The model under review builds one solid part; all positions refer to its coordinate system, in mm. Round coordinates to 2 decimals unless told otherwise and drop trailing zeros. Loops run counter-clockwise (first coordinate to the right, second up) from the corner with the lowest first, then second, coordinate; pieces in that order, holes last. Notation, with made-up numbers: (-37.5, 45.25) -> (-26.5, 45.25) arc R25 cw to (-26.5, 83.25) -> close; hole circle Ø1 at (28, 14.5). An arc over 180 degrees is marked (long way). Use a Markdown table: item, result. Add a question column.
1) Consider section A-A on z = 76.5. Give the boundary of the cut face in (x, y), plus the area to 3 significant figures.
2) Consider section C-C on x = -79. Give the boundary of the cut face in (y, z), plus the area to 3 significant figures.
3) Consider section B-B on y = 0.8. State how many separate pieces and enclosed holes the cut face has, plus the area to 3 significant figures.
4) Wall thickness on probe 1 along X at (y, z) = (1.95, -115.5); probe 2 along Z at (x, y) = (101.6, 2.7); probe 3 along X at (y, z) = (4.45, 19): over which ranges is each line inside the solid? List them lowest first.
5) Insertion check: pin 1 (1 mm diameter, centred on y = 3, z = 3, fed in from -X); pin 2 (2.5 mm diameter, centred on y = 3, z = -164.5, fed in from +X); pin 3 (2.5 mm diameter, centred on y = 3.5, z = -164, fed in from -X). Each pin has a flat end and moves straight along its axis. Give the tip position at first contact, or say it passes through.
from build123d import *

# Parameters (mm, degrees)
SKETCH1_R           = 177
SKETCH1_R_2         = 1.6
SKETCH1_R_3         = 2.2479
SKETCH1_R_4         = 2.000000064
SKETCH1_R_5         = 1.3
SKETCH1_R_6         = 1.29999994
SKETCH1_W           = 6.15
SKETCH1_H           = 6.15
SKETCH1_W_2         = 30
SKETCH1_H_2         = 80
SKETCH1_W_3         = 6.35
SKETCH1_H_3         = 3.175
BOSS_EXTRUDE1_DEPTH = 4.7625
SKETCH2_R           = 1.599999975
CUT_EXTRUDE1_DEPTH  = 251.361102023
SKETCH3_R           = 1.3
SKETCH3_R_2         = 1.29999994
SKETCH3_W           = 6.15
SKETCH3_H           = 6.15
CUT_EXTRUDE2_DEPTH  = 251.361102023


with BuildPart() as part:
    # Sketch1 → Boss-Extrude1 (new body)
    with BuildSketch(Plane(origin=(0, 0, 0), x_dir=(1, 0, 0), z_dir=(0, 1, 0))):
        with Locations(Location((0, 0, 0), (0, 0, 90))):
            Circle(SKETCH1_R)
        with Locations(Location((-150.65, 25.4, 0), (0, 0, 90))):
            Circle(SKETCH1_R_2, mode=Mode.SUBTRACT)
        with Locations(Location((-150.65, -25.4, 0), (0, 0, 90))):
            Circle(SKETCH1_R_2, mode=Mode.SUBTRACT)
        with Locations(Location((150.65, 25.4, 0), (0, 0, 90))):
            Circle(SKETCH1_R_2, mode=Mode.SUBTRACT)
        with Locations(Location((150.65, -25.4, 0), (0, 0, 90))):
            Circle(SKETCH1_R_2, mode=Mode.SUBTRACT)
        with Locations(Location((-107.95, 25.4, 0), (0, 0, 90))):
            Circle(SKETCH1_R_2, mode=Mode.SUBTRACT)
        with Locations(Location((-107.95, -25.4, 0), (0, 0, 90))):
            Circle(SKETCH1_R_2, mode=Mode.SUBTRACT)
        with Locations(Location((107.95, 25.4, 0), (0, 0, 90))):
            Circle(SKETCH1_R_2, mode=Mode.SUBTRACT)
        with Locations(Location((107.95, -25.4, 0), (0, 0, 90))):
            Circle(SKETCH1_R_2, mode=Mode.SUBTRACT)
        with Locations(Location((-53.7, 114.3, 0), (0, 0, 90))):
            Circle(SKETCH1_R_2, mode=Mode.SUBTRACT)
        with Locations(Location((38.8, 114.3, 0), (0, 0, 90))):
            Circle(SKETCH1_R_2, mode=Mode.SUBTRACT)
        with Locations(Location((-53.7, 35.8, 0), (0, 0, 90))):
            Circle(SKETCH1_R_2, mode=Mode.SUBTRACT)
        with Locations(Location((38.8, 35.8, 0), (0, 0, 90))):
            Circle(SKETCH1_R_2, mode=Mode.SUBTRACT)
        with Locations(Location((-101.6, -101.6, 0), (0, 0, 90))):
            Circle(SKETCH1_R_3, mode=Mode.SUBTRACT)
        with Locations(Location((101.6, -101.6, 0), (0, 0, 90))):
            Circle(SKETCH1_R_3, mode=Mode.SUBTRACT)
        with Locations(Location((-101.6, 101.6, 0), (0, 0, 90))):
            Circle(SKETCH1_R_3, mode=Mode.SUBTRACT)
        with Locations(Location((101.6, 101.6, 0), (0, 0, 90))):
            Circle(SKETCH1_R_3, mode=Mode.SUBTRACT)
        with Locations(Location((-20, -142.687006289, 0), (0, 0, 90))):
            Circle(SKETCH1_R_4, mode=Mode.SUBTRACT)
        with Locations(Location((20, -142.687006289, 0), (0, 0, 90))):
            Circle(SKETCH1_R_4, mode=Mode.SUBTRACT)
        with Locations(Location((-20, 151.719279026, 0), (0, 0, 90))):
            Circle(SKETCH1_R_4, mode=Mode.SUBTRACT)
        with Locations(Location((20, 151.719279026, 0), (0, 0, 90))):
            Circle(SKETCH1_R_4, mode=Mode.SUBTRACT)
        with Locations(Location((-10.125, -171.45, 0), (0, 0, 90))):
            Circle(SKETCH1_R_5, mode=Mode.SUBTRACT)
        with Locations(Location((10.125, -171.45, 0), (0, 0, 90))):
            Circle(SKETCH1_R_6, mode=Mode.SUBTRACT)
        with Locations(Location((171.45, -10.125, 0), (0, 0, 90))):
            Circle(SKETCH1_R_5, mode=Mode.SUBTRACT)
        with Locations(Location((171.45, 10.125, 0), (0, 0, 90))):
            Circle(SKETCH1_R_5, mode=Mode.SUBTRACT)
        with Locations(Location((-171.45, -10.125, 0), (0, 0, 90))):
            Circle(SKETCH1_R_5, mode=Mode.SUBTRACT)
        with Locations(Location((-171.45, 10.125, 0), (0, 0, 90))):
            Circle(SKETCH1_R_5, mode=Mode.SUBTRACT)
        with Locations((171.45, 4.26)):
            Rectangle(SKETCH1_W, SKETCH1_H, mode=Mode.SUBTRACT)
        with Locations((-129.3, 0)):
            Rectangle(SKETCH1_W_2, SKETCH1_H_2, mode=Mode.SUBTRACT)
        with Locations((129.3, 0)):
            Rectangle(SKETCH1_W_2, SKETCH1_H_2, mode=Mode.SUBTRACT)
        with Locations((4.26, -171.45)):
            Rectangle(SKETCH1_W, SKETCH1_H, mode=Mode.SUBTRACT)
        with Locations((-171.45, 4.26)):
            Rectangle(SKETCH1_W, SKETCH1_H, mode=Mode.SUBTRACT)
        with Locations((-18.119952608, 164.452014647)):
            Rectangle(SKETCH1_W_3, SKETCH1_H_3, mode=Mode.SUBTRACT)
        with Locations((-30.819952608, 164.452014647)):
            Rectangle(SKETCH1_W_3, SKETCH1_H_3, mode=Mode.SUBTRACT)
        with Locations((-5.419952608, 164.452014647)):
            Rectangle(SKETCH1_W_3, SKETCH1_H_3, mode=Mode.SUBTRACT)
        with Locations((7.280047392, 164.452014647)):
            Rectangle(SKETCH1_W_3, SKETCH1_H_3, mode=Mode.SUBTRACT)
        with Locations((19.980047392, 164.452014647)):
            Rectangle(SKETCH1_W_3, SKETCH1_H_3, mode=Mode.SUBTRACT)
        with Locations((32.680047392, 164.452014647)):
            Rectangle(SKETCH1_W_3, SKETCH1_H_3, mode=Mode.SUBTRACT)
    extrude(amount=BOSS_EXTRUDE1_DEPTH)

    # Sketch2 → Cut-Extrude1 (cut, through all)
    with BuildSketch(Plane(origin=(0, 4.7625, 0), x_dir=(1, 0, 0), z_dir=(0, 1, 0))):
        with Locations(Location((21.59, 21.689999946, 0), (0, 0, 270))):
            Circle(SKETCH2_R)
        with Locations(Location((21.59, -21.690000054, 0), (0, 0, 270))):
            Circle(SKETCH2_R)
        with Locations(Location((72.470000006, -21.690000054, 0), (0, 0, 270))):
            Circle(SKETCH2_R)
        with Locations(Location((72.470000006, 21.689999946, 0), (0, 0, 270))):
            Circle(SKETCH2_R)
        with Locations(Location((-72.470000006, 21.689999946, 0), (0, 0, 270))):
            Circle(SKETCH2_R)
        with Locations(Location((-72.470000006, -21.690000054, 0), (0, 0, 270))):
            Circle(SKETCH2_R)
        with Locations(Location((-21.59, -21.690000054, 0), (0, 0, 270))):
            Circle(SKETCH2_R)
        with Locations(Location((-21.59, 21.689999946, 0), (0, 0, 270))):
            Circle(SKETCH2_R)
    extrude(amount=-CUT_EXTRUDE1_DEPTH, mode=Mode.SUBTRACT)

    # Sketch3 → Cut-Extrude2 (cut, through all)
    with BuildSketch(Plane(origin=(0, 4.7625, 0), x_dir=(1, 0, 0), z_dir=(0, 1, 0))):
        with Locations(Location((-8.77, 171.169, 0), (0, 0, 270))):
            Circle(SKETCH3_R)
        with Locations(Location((11.48, 171.169, 0), (0, 0, 270))):
            Circle(SKETCH3_R_2)
        with Locations((5.615, 171.169)):
            Rectangle(SKETCH3_W, SKETCH3_H)
    extrude(amount=-CUT_EXTRUDE2_DEPTH, mode=Mode.SUBTRACT)


solid = part.part
Result set:
| question | item | result |
|---|---|---|
| 1 | outline | (-159.61, 0) -> (159.61, 0) -> (159.61, 4.76) -> (-159.61, 4.76) -> close |
| 1 | area | 1,520 mm2 |
| 2 | outline | (0, -158.39) -> (4.76, -158.39) -> (4.76, 158.39) -> (0, 158.39) -> close |
| 2 | area | 1,510 mm2 |
| 3 | separate pieces | 1 |
| 3 | enclosed holes | 48 |
| 3 | area | 93,000 mm2 |
| 4 | probe 1 | -134.12 to -54.76, -52.64 to 37.74, 39.86 to 134.12 |
| 4 | probe 2 | -144.94 to -103.85, -99.35 to 99.35, 103.85 to 144.94 |
| 4 | probe 3 | -175.98 to -144.3, -114.3 to 114.3, 144.3 to 175.98 |
| 5 | pin 1 | x = -176.98 |
| 5 | pin 2 | x = 68.4 |
| 5 | pin 3 | x = -69.58 |
